Geometry check sheet. Reference: the model listing, model coordinates, mm. A direction names the side the tool comes from. Round coordinates to 2 decimals unless told otherwise and drop trailing zeros. Loops run counter-clockwise (first coordinate to the right, second up) from the corner with the lowest first, then second, coordinate; pieces in that order, holes last. Notation, with made-up numbers: (-4.75, 60) -> (44.25, 60) arc R25 ccw to (44.25, 76) -> close; hole circle Ø10 at (63, 55.5). An arc over 180 degrees is marked (long way). Use one line per item in the form item = value.
from build123d import *

# Parameters (mm, degrees)
BOSS_EXTRUDE1_DEPTH = 6.35
SKETCH2_R           = 28.956
SKETCH2_R_2         = 4.318
CUT_EXTRUDE1_DEPTH  = 129.84998677


with BuildPart() as part:
    # Sketch1 → Boss-Extrude1 (new body)
    with BuildSketch(Plane.XY):
        with BuildLine():
            Line((2.85403164, 83.616306594), (5.563187423, 90.860395533))
            Line((5.563187423, 90.860395533), (11.732789539, 90.271269961))
            Line((11.732789539, 90.271269961), (13.022034501, 82.645380043))
            ThreePointArc((13.022034501, 82.645380043), (15.833705359, 82.153064456), (18.626945642, 81.565121964))
            Line((18.626945642, 81.565121964), (22.658096297, 88.165589676))
            Line((22.658096297, 88.165589676), (28.604712917, 86.419505493))
            Line((28.604712917, 86.419505493), (28.427450387, 78.687434127))
            ThreePointArc((28.427450387, 78.687434127), (31.095139353, 77.671903116), (33.726633297, 76.565961311))
            Line((33.726633297, 76.565961311), (38.934082535, 82.284249695))
            Line((38.934082535, 82.284249695), (44.442787442, 79.444314933))
            Line((44.442787442, 79.444314933), (42.805424149, 71.885519323))
            ThreePointArc((42.805424149, 71.885519323), (45.232713992, 70.383476824), (47.60735255, 68.799507325))
            Line((47.60735255, 68.799507325), (53.802889589, 73.42894254))
            Line((53.802889589, 73.42894254), (58.674583834, 69.597799841))
            Line((58.674583834, 69.597799841), (55.636298354, 62.485474556))
            ThreePointArc((55.636298354, 62.485474556), (57.735460496, 60.551208298), (59.767418042, 58.546459889))
            Line((59.767418042, 58.546459889), (66.727120031, 61.919722085))
            Line((66.727120031, 61.919722085), (70.785727891, 57.235838927))
            Line((70.785727891, 57.235838927), (66.456331777, 50.827041933))
            ThreePointArc((66.456331777, 50.827041933), (68.151497028, 48.530461339), (69.767333324, 46.177390852))
            Line((69.767333324, 46.177390852), (77.239658499, 48.172561544))
            Line((77.239658499, 48.172561544), (80.338491312, 42.805225668))
            Line((80.338491312, 42.805225668), (74.87446022, 37.331587587))
            ThreePointArc((74.87446022, 37.331587587), (76.104360891, 34.755697063), (77.245675402, 32.139350595))
            Line((77.245675402, 32.139350595), (84.960554463, 32.684319115))
            Line((84.960554463, 32.684319115), (86.987612337, 26.827520026))
            Line((86.987612337, 26.827520026), (80.586430587, 22.486872398))
            ThreePointArc((80.586430587, 22.486872398), (81.306614864, 19.724771339), (81.93215751, 16.939710469))
            Line((81.93215751, 16.939710469), (89.610754626, 16.014780236))
            Line((89.610754626, 16.014780236), (90.492774408, 9.880197911))
            Line((90.492774408, 9.880197911), (83.385797386, 6.829423052))
            ThreePointArc((83.385797386, 6.829423052), (83.570235933, 3.980940987), (83.657397973, 1.127825071))
            Line((83.657397973, 1.127825071), (91.022188639, -1.233574527))
            Line((91.022188639, -1.233574527), (90.727291835, -7.424220299))
            Line((90.727291835, -7.424220299), (83.171384209, -9.074859436))
            ThreePointArc((83.171384209, -9.074859436), (82.813410935, -11.906770944), (82.359042106, -14.724822863))
            Line((82.359042106, -14.724822863), (89.143843598, -18.437344692))
            Line((89.143843598, -18.437344692), (87.682688548, -24.460307843))
            Line((87.682688548, -24.460307843), (79.950940505, -24.651152861))
            ThreePointArc((79.950940505, -24.651152861), (79.063493498, -27.364141151), (78.084015873, -30.045277335))
            Line((78.084015873, -30.045277335), (84.043607787, -34.974741183))
            Line((84.043607787, -34.974741183), (81.469004441, -40.612336132))
            Line((81.469004441, -40.612336132), (73.840861501, -39.336489393))
            ThreePointArc((73.840861501, -39.336489393), (72.456015408, -41.8325), (70.986829861, -44.279817201))
            Line((70.986829861, -44.279817201), (75.905817018, -50.248059401))
            Line((75.905817018, -50.248059401), (72.310818249, -55.296528778))
            Line((72.310818249, -55.296528778), (65.061981372, -52.600102708))
            ThreePointArc((65.061981372, -52.600102708), (63.229788138, -54.788923305), (61.323994863, -56.913969103))
            Line((61.323994863, -56.913969103), (65.024592251, -63.705281833))
            Line((65.024592251, -63.705281833), (60.539130681, -67.982160801))
            Line((60.539130681, -67.982160801), (53.931591719, -63.962611264))
            ThreePointArc((53.931591719, -63.962611264), (51.718271582, -65.765132172), (49.444750912, -67.491101874))
            Line((49.444750912, -67.491101874), (51.7932093, -74.860029396))
            Line((51.7932093, -74.860029396), (46.579401197, -78.210740406))
            Line((46.579401197, -78.210740406), (40.851973824, -73.013344395))
            ThreePointArc((40.851973824, -73.013344395), (38.33752194, -74.364417812), (35.778444837, -75.628930378))
            Line((35.778444837, -75.628930378), (36.689884819, -83.309140451))
            Line((36.689884819, -83.309140451), (30.936170793, -85.612580077))
            Line((30.936170793, -85.612580077), (26.295859156, -79.425185025))
            ThreePointArc((26.295859156, -79.425185025), (23.571154368, -80.275979637), (20.819012545, -81.033332288))
            Line((20.819012545, -81.033332288), (20.260492306, -88.747242111))
            Line((20.260492306, -88.747242111), (14.174826572, -89.920158042))
            Line((14.174826572, -89.920158042), (10.789343625, -82.966392528))
            ThreePointArc((10.789343625, -82.966392528), (7.952863863, -83.286158402), (5.107126896, -83.508978439))
            Line((5.107126896, -83.508978439), (3.098832813, -90.977787212))
            Line((3.098832813, -90.977787212), (-3.098832812, -90.977787212))
            Line((-3.098832812, -90.977787212), (-5.107126896, -83.508978439))
            ThreePointArc((-5.107126896, -83.508978439), (-7.952863863, -83.286158402), (-10.789343625, -82.966392528))
            Line((-10.789343625, -82.966392528), (-14.174826572, -89.920158042))
            Line((-14.174826572, -89.920158042), (-20.260492306, -88.747242111))
            Line((-20.260492306, -88.747242111), (-20.819012545, -81.033332288))
            ThreePointArc((-20.819012545, -81.033332288), (-23.571154368, -80.275979637), (-26.295859156, -79.425185025))
            Line((-26.295859156, -79.425185025), (-30.936170793, -85.612580077))
            Line((-30.936170793, -85.612580077), (-36.689884818, -83.309140451))
            Line((-36.689884818, -83.309140451), (-35.778444837, -75.628930378))
            ThreePointArc((-35.778444837, -75.628930378), (-38.33752194, -74.364417812), (-40.851973824, -73.013344395))
            Line((-40.851973824, -73.013344395), (-46.579401197, -78.210740406))
            Line((-46.579401197, -78.210740406), (-51.7932093, -74.860029396))
            Line((-51.7932093, -74.860029396), (-49.444750912, -67.491101875))
            ThreePointArc((-49.444750912, -67.491101875), (-51.718271582, -65.765132172), (-53.931591719, -63.962611264))
            Line((-53.931591719, -63.962611264), (-60.539130681, -67.982160801))
            Line((-60.539130681, -67.982160801), (-65.024592251, -63.705281833))
            Line((-65.024592251, -63.705281833), (-61.323994863, -56.913969103))
            ThreePointArc((-61.323994863, -56.913969103), (-63.229788138, -54.788923306), (-65.061981372, -52.600102708))
            Line((-65.061981372, -52.600102708), (-72.310818249, -55.296528778))
            Line((-72.310818249, -55.296528778), (-75.905817018, -50.248059401))
            Line((-75.905817018, -50.248059401), (-70.986829861, -44.279817201))
            ThreePointArc((-70.986829861, -44.279817201), (-72.456015408, -41.8325), (-73.840861501, -39.336489393))
            Line((-73.840861501, -39.336489393), (-81.469004441, -40.612336132))
            Line((-81.469004441, -40.612336132), (-84.043607787, -34.974741183))
            Line((-84.043607787, -34.974741183), (-78.084015873, -30.045277335))
            ThreePointArc((-78.084015873, -30.045277335), (-79.063493498, -27.364141151), (-79.950940505, -24.651152861))
            Line((-79.950940505, -24.651152861), (-87.682688547, -24.460307844))
            Line((-87.682688547, -24.460307844), (-89.143843598, -18.437344693))
            Line((-89.143843598, -18.437344693), (-82.359042106, -14.724822863))
            ThreePointArc((-82.359042106, -14.724822863), (-82.813410935, -11.906770944), (-83.171384209, -9.074859436))
            Line((-83.171384209, -9.074859436), (-90.727291835, -7.424220299))
            Line((-90.727291835, -7.424220299), (-91.022188639, -1.233574527))
            Line((-91.022188639, -1.233574527), (-83.657397973, 1.127825071))
            ThreePointArc((-83.657397973, 1.127825071), (-83.570235933, 3.980940987), (-83.385797386, 6.829423052))
            Line((-83.385797386, 6.829423052), (-90.492774407, 9.880197911))
            Line((-90.492774407, 9.880197911), (-89.610754626, 16.014780236))
            Line((-89.610754626, 16.014780236), (-81.93215751, 16.939710469))
            ThreePointArc((-81.93215751, 16.939710469), (-81.306614864, 19.724771339), (-80.586430587, 22.486872398))
            Line((-80.586430587, 22.486872398), (-86.987612336, 26.827520026))
            Line((-86.987612336, 26.827520026), (-84.960554463, 32.684319115))
            Line((-84.960554463, 32.684319115), (-77.245675402, 32.139350595))
            ThreePointArc((-77.245675402, 32.139350595), (-76.104360891, 34.755697063), (-74.87446022, 37.331587587))
            Line((-74.87446022, 37.331587587), (-80.338491312, 42.805225668))
            Line((-80.338491312, 42.805225668), (-77.239658499, 48.172561544))
            Line((-77.239658499, 48.172561544), (-69.767333324, 46.177390852))
            ThreePointArc((-69.767333324, 46.177390852), (-68.151497028, 48.530461339), (-66.456331777, 50.827041933))
            Line((-66.456331777, 50.827041933), (-70.785727891, 57.235838927))
            Line((-70.785727891, 57.235838927), (-66.727120031, 61.919722085))
            Line((-66.727120031, 61.919722085), (-59.767418042, 58.546459889))
            ThreePointArc((-59.767418042, 58.546459889), (-57.735460496, 60.551208298), (-55.636298354, 62.485474556))
            Line((-55.636298354, 62.485474556), (-58.674583834, 69.597799841))
            Line((-58.674583834, 69.597799841), (-53.802889589, 73.42894254))
            Line((-53.802889589, 73.42894254), (-47.60735255, 68.799507325))
            ThreePointArc((-47.60735255, 68.799507325), (-45.232713992, 70.383476824), (-42.805424149, 71.885519323))
            Line((-42.805424149, 71.885519323), (-44.442787442, 79.444314933))
            Line((-44.442787442, 79.444314933), (-38.934082535, 82.284249695))
            Line((-38.934082535, 82.284249695), (-33.726633297, 76.565961311))
            ThreePointArc((-33.726633297, 76.565961311), (-31.095139353, 77.671903116), (-28.427450387, 78.687434127))
            Line((-28.427450387, 78.687434127), (-28.604712917, 86.419505493))
            Line((-28.604712917, 86.419505493), (-22.658096297, 88.165589676))
            Line((-22.658096297, 88.165589676), (-18.626945642, 81.565121964))
            ThreePointArc((-18.626945642, 81.565121964), (-15.833705359, 82.153064456), (-13.022034501, 82.645380043))
            Line((-13.022034501, 82.645380043), (-11.732789539, 90.271269961))
            Line((-11.732789539, 90.271269961), (-5.563187423, 90.860395533))
            Line((-5.563187423, 90.860395533), (-2.85403164, 83.616306594))
            ThreePointArc((-2.85403164, 83.616306594), (0, 83.665), (2.85403164, 83.616306594))
        make_face()
    extrude(amount=BOSS_EXTRUDE1_DEPTH)

    # Sketch2 → Cut-Extrude1 (cut, through all)
    with BuildSketch(Plane(origin=(0, 0, 0), x_dir=(-1, 0, 0), z_dir=(0, 0, -1))):
        Circle(SKETCH2_R)
        with Locations((0, 45.0088)):
            Circle(SKETCH2_R_2)
        with Locations((31.826027693, 31.826027693)):
            Circle(SKETCH2_R_2)
        with Locations((45.0088, 0)):
            Circle(SKETCH2_R_2)
        with Locations((31.826027693, -31.826027693)):
            Circle(SKETCH2_R_2)
        with Locations((0, -45.0088)):
            Circle(SKETCH2_R_2)
        with Locations((-31.826027693, -31.826027693)):
            Circle(SKETCH2_R_2)
        with Locations((-45.0088, 0)):
            Circle(SKETCH2_R_2)
        with Locations((-31.826027693, 31.826027693)):
            Circle(SKETCH2_R_2)
    extrude(amount=-CUT_EXTRUDE1_DEPTH, mode=Mode.SUBTRACT)


solid = part.part
1. Mould release check, pull along Y, two halves, no side actions. Record for faces 1 (the flat face through (-85.99, 29.71, 3.13)), 2 (the cylindrical face through (-28.399, -34.453, 3.131)), 3 (the flat face through (28.648, -82.562, 3.131)): released by +Y, released by -Y, zero draft, split by the parting line, or undercut.
Return value:
face_1 = released by +Y
face_2 = undercut
face_3 = released by -Y
2. Section check A-A (x = 0). Record the boundary of the cut face in (y, z) (3 decimals).
Return value:
outline = (-90.978, 0) -> (-49.327, 0) -> (-49.327, 6.35) -> (-90.978, 6.35) -> close; (-40.691, 0) -> (-28.956, 0) -> (-28.956, 6.35) -> (-40.691, 6.35) -> close; (28.956, 0) -> (40.691, 0) -> (40.691, 6.35) -> (28.956, 6.35) -> close; (49.327, 0) -> (83.665, 0) -> (83.665, 6.35) -> (49.327, 6.35) -> close
3. Section check C-C (z = 3). Count the separate pieces of the cut face and the enclosed holes in it, then the cut area to 3 significant figures.
Return value:
separate_pieces = 1
enclosed_holes = 9
area = 20,900 mm2
4. Material ranges on line 1 along Y through (x, z) = (0, 4.75) (3 decimals); line 2 along X through (y, z) = (71, 0.5); line 3 along X through (y, z) = (5, 2.75), recorded low to high.
Return value:
line_1 = -90.978 to -49.327, -40.691 to -28.956, 28.956 to 40.691, 49.327 to 83.665
line_2 = -56.89 to -50.55, -44.26 to 44.26, 50.55 to 56.89
line_3 = -83.52 to -28.52, 28.52 to 83.52
5. Section check B-B (y = -21.5). Record the boundary of the cut face in (x, z).
Return value:
outline = (-88.4, 0) -> (-19.4, 0) -> (-19.4, 6.35) -> (-88.4, 6.35) -> close; (19.4, 0) -> (88.4, 0) -> (88.4, 6.35) -> (19.4, 6.35) -> close
6. Tool access check on faces 4 (the cylindrical face through (-7.91, -83.29, 3.13)), 5 (the flat face through (-57.134, 65.992, 3.131)), 6 (the cylindrical face through (51.75, -65.74, 3.13)). Record the directions out of +Z, -Z, +X, -X, +Y, -Y that give a thin tool (end or side, any length) a straight path to the whole face; none if there is none.
Return value:
face_4 = +Z, -Z, -Y
face_5 = +Z, -Z, -X
face_6 = +Z, -Z
7. Section check D-D (y = 65.5). Record the boundary of the cut face in (x, z).
Return value:
outline = (-56.92, 0) -> (56.92, 0) -> (56.92, 6.35) -> (-56.92, 6.35) -> close
8. Gauge pin test, flat ends, axial feed: pin 1 (14 mm diameter, centred on x = 0, y = 45.01, fed in from +Z); pin 2 (1.5 mm diameter, centred on y = -32.5, z = 1, fed in from -X); pin 3 (1 mm diameter, centred on y = -23.5, z = 2.5, fed in from -X); pin 4 (1.5 mm diameter, centred on x = -62, z = 4, fed in from +Y). Record the tip position at first contact, or that the pin passes through.
Return value:
pin_1 = 6.35
pin_2 = -81.96
pin_3 = -88.04
pin_4 = 59.99
